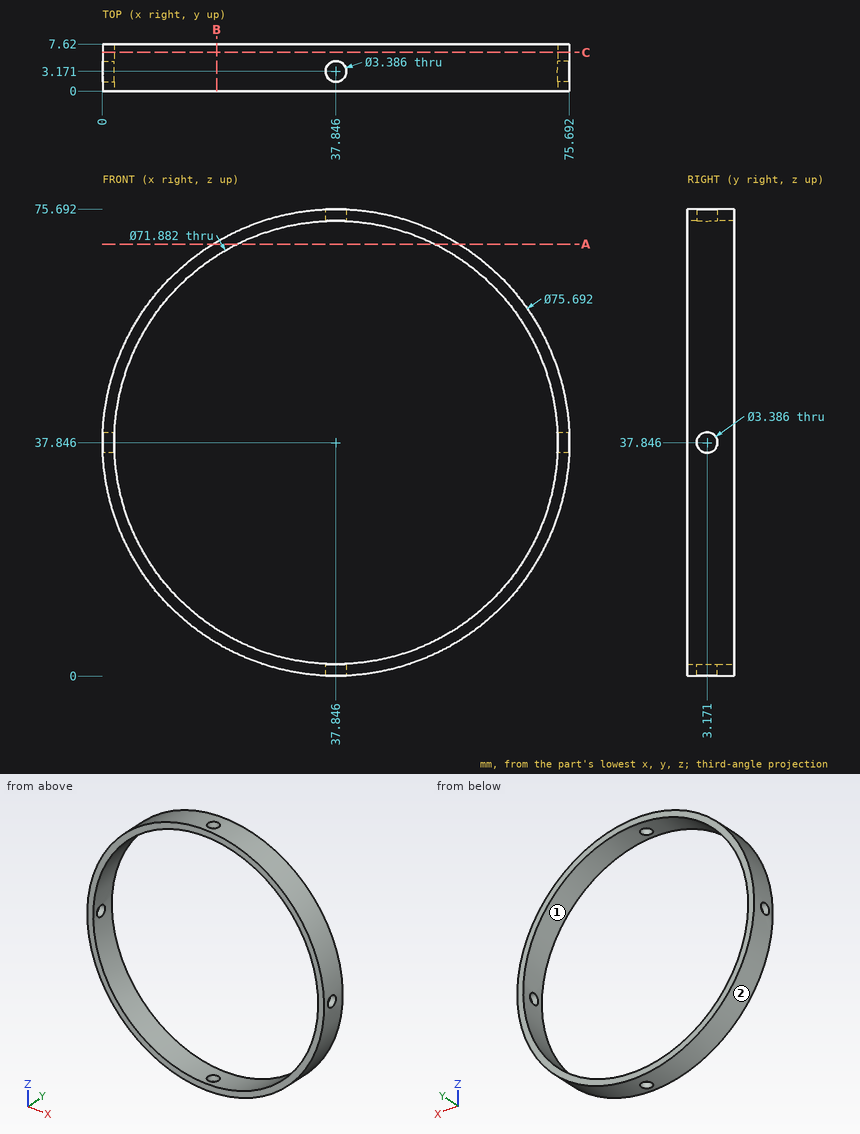
Input: dimensioned drawing with shaded views. Units: mm. Origin: part minimum x, y, z. Round coordinates to 2 decimals unless told otherwise and drop trailing zeros. Loops run counter-clockwise (first coordinate to the right, second up) from the corner with the lowest first, then second, coordinate; pieces in that order, holes last. Notation, with made-up numbers: (-27, 56) -> (14, 56) arc R31 cw to (14, 87) -> close; hole circle Ø10 at (-24.75, 57). An arc over 180 degrees is marked (long way). Use one line per item in the form item = value. Start each with the question number.
1) Section C-C on y = 6.25. Output: boundary loops of the cut face in (x, z) (1 decimal).
2) First-contact query: P1, Ø3, axis at y = 5.5, z = 61, coming from the -X side; P2, Ø1.5, axis at x = 20.5, y = 3.5, coming from the +Z side; P3, Ø1, axis at x = 19.5, y = 2, coming from the -Z side; P4, Ø2, axis at y = 3.17, z = 37.85, coming from the -X side. Flat tips, straight axial feed; report the tip coordinate or a pass-through.
3) Section B-B on x = 18.5. Output: boundary loops of the cut face in (y, z).
4) Section A-A on z = 70. Output: boundary loops of the cut face in (x, y) (1 decimal).
5) Draft query along Z for the marked faces 1 and 2. Return one class per face: released by +Z, released by -Z, zero draft, split by the parting line, or undercut.
6) Line query: L1, parallel to X at y = 3.25, z = 66 (1 decimal); L2, parallel to X at y = 6, z = 34; L3, parallel to Z at x = 49.5, y = 0.5 (1 decimal). Output: solid intervals per line, ascending.
Response:
q1.outline = circle Ø75.7 at (37.8, 37.8); hole circle Ø71.9 at (37.8, 37.8)
q2.P1 = 6.81
q2.P2 = 71.86
q2.P3 = 4.47
q2.P4 = through
q3.outline = (0, 5.32) -> (7.62, 5.32) -> (7.62, 7.56) -> (0, 7.56) -> close; (0, 68.14) -> (7.62, 68.14) -> (7.62, 70.37) -> (0, 70.37) -> close
q4.outline = (17.9, 0) -> (21.8, 0) -> (21.8, 7.6) -> (17.9, 7.6) -> close; (53.9, 0) -> (57.8, 0) -> (57.8, 7.6) -> (53.9, 7.6) -> close
q5.face_1 = undercut
q5.face_2 = split by the parting line
q6.L1 = 12.6 to 15.5, 60.2 to 63.1
q6.L2 = 0.2 to 2.11, 73.58 to 75.5
q6.L3 = 1.8 to 3.8, 71.8 to 73.9
